The figure shows three views and two pictorial views of one solid part (mm, origin at its lowest corner). Answer the questions. Give positions to 0.01 mm unless a question says otherwise; leave off trailing zeros. Loops run counter-clockwise (first coordinate to the right, second up) from the corner with the lowest first, then second, coordinate; pieces in that order, holes last. Notation, with made-up numbers: M -32,78 L 12,78 A7 ccw 12,88 Z; hole C 11.25,76 d2. An arc over 180 degrees is marked long. Answer in a Markdown table with one row per item. Add a question column.
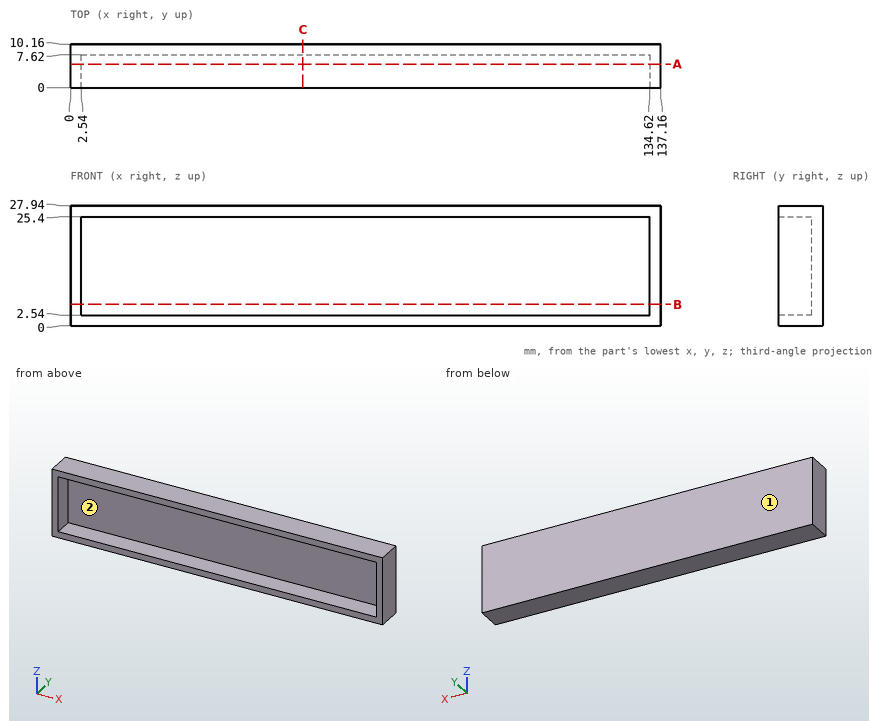
(1) Consider line 1 along X through (y, z) = (3.25, 3.75); line 2 along Z through (x, y) = (102, 3.75); line 3 along Y through (x, z) = (64, 20.25). Determine where each line is inside the solid, lowest interval first. Write a range as from..to.
(2) The mould has two halves that part along Z. Classify the marked faces 1 and 2: pulls with the +Z half, pulls with the -Z half, needs draft (parallel to the pull), parting line crosses it, or undercut.
(3) This flat-tipped pin is pushed along its axis until it touches: P1, Ø1.5, axis at x = 31, z = 22, coming from the -Y side. Where does it stop, or does it pass through?
(4) Section A-A, the plane y = 5.5 is taken. Determine the outline of the cut face in (x, z), and give its area (3 significant figures).
(5) Section B-B, the plane z = 5 is taken. Determine the outline of the cut face in (x, y).
(6) Section C-C, the plane x = 54 is taken. Determine the outline of the cut face in (y, z).
Numbers:
| question | item | result |
|---|---|---|
| 1 | line 1 | x = 0..2.54, 134.62..137.16 |
| 1 | line 2 | z = 0..2.54, 25.4..27.94 |
| 1 | line 3 | y = 7.62..10.16 |
| 2 | face 1 | needs draft |
| 2 | face 2 | undercut |
| 3 | P1 | stops at y = 7.62 |
| 4 | outline | M 0,0 L 137.16,0 L 137.16,27.94 L 0,27.94 Z; hole M 2.54,2.54 L 134.62,2.54 L 134.62,25.4 L 2.54,25.4 Z |
| 4 | area | 813 mm² |
| 5 | outline | M 0,0 L 2.54,0 L 2.54,7.62 L 134.62,7.62 L 134.62,0 L 137.16,0 L 137.16,10.16 L 0,10.16 Z |
| 6 | outline | M 0,0 L 10.16,0 L 10.16,27.94 L 0,27.94 L 0,25.4 L 7.62,25.4 L 7.62,2.54 L 0,2.54 Z |
